```python
from build123d import *

# Parameters (mm, degrees)
EXTRUDE_3_DEPTH     = 5
SKETCH_1_R          = 9.79888
CUT_EXTRUDE_1_DEPTH = 1.65
SKETCH_1_9_R        = 3.15
SKETCH_3_8_R        = 1.65
SKETCH_3_9_R        = 1.648905
SKETCH_3_9_R_2      = 1.65
CUT_EXTRUDE_2_DEPTH = 5
SKETCH_10_R         = 11.19888
CUT_EXTRUDE_3_DEPTH = 3.35
EXTRUDE_4_DEPTH     = 28
EXTRUDE_5_DEPTH     = 2
EXTRUDE_6_DEPTH     = 28


with BuildPart() as part:
    # Sketch 7 → Extrude 3 (new body)
    with BuildSketch(Plane.XY):
        with BuildLine():
            Line((14, 14), (-14, 14))
            Line((-14, 14), (-14, 0))
            ThreePointArc((-14, 0), (-12.934313455, -5.357568053), (-9.899494937, -9.899494937))
            Line((-9.899494937, -9.899494937), (-2.121320344, -17.67766953))
            ThreePointArc((-2.121320344, -17.67766953), (0.000404905, -18.556181469), (2.121892965, -17.677096908))
            Line((2.121892965, -17.677096908), (9.899494937, -9.899494937))
            ThreePointArc((9.899494937, -9.899494937), (12.934313455, -5.357568053), (14, 0))
            Line((14, 0), (14, 14))
        make_face()
    extrude(amount=-EXTRUDE_3_DEPTH)

    # Sketch 1 → Cut-Extrude 1 (cut)
    with BuildSketch(Plane.XY):
        Circle(SKETCH_1_R)
    extrude(amount=-CUT_EXTRUDE_1_DEPTH, mode=Mode.SUBTRACT)

    # Loft 1: read off the stored shape, not the designer's step
    # Loft 1 outline → Loft 1 (revolve, cut)
    with BuildSketch(Plane(origin=(10.6066, 10.606603436, 0), x_dir=(1, 0, 0), z_dir=(0, -1, 0))):
        Polygon((0, 0), (0, -1.5), (1.648905, -1.5), (3.15, 0), align=None)
    revolve(axis=Axis((10.6066, 10.606603436, 0), (0, 0, 1)), mode=Mode.SUBTRACT)

    # Loft 2: read off the stored shape, not the designer's step
    # Loft 2: loft between two sections, ruled curve by curve
    loft_2_from = [
        Edge.make_bspline([(-8.058196468, 12.45812698, 0), (-4.355149378, 7.361319916, 0), (-9.451956443, 3.658272826, 0), (-13.155003532, 8.755079891, 0), (-16.858050622, 13.851886955, 0), (-11.761243557, 17.554934045, 0), (-8.058196468, 12.45812698, 0)], [0, 0, 0, 0, 0.5, 0.5, 0.5, 1, 1, 1, 1], 3, [1, 0.333333333, 0.333333333, 1, 0.333333333, 0.333333333, 1]),
    ]
    loft_2_to = [
        Edge.make_bspline([(-9.518492924, 11.845518562, -1.5), (-7.040662671, 9.669304411, -1.5), (-9.216876823, 7.191474158, -1.5), (-11.694707076, 9.367688309, -1.5), (-14.172537329, 11.543902461, -1.5), (-11.996323177, 14.021732714, -1.5), (-9.518492924, 11.845518562, -1.5)], [0, 0, 0, 0, 0.5, 0.5, 0.5, 1, 1, 1, 1], 3, [1, 0.333333333, 0.333333333, 1, 0.333333333, 0.333333333, 1]),
    ]
    loft_2 = Solid(Shell([*[Face.make_surface_from_curves(loft_2_from[k], loft_2_to[k]) for k in range(1)], Face(Wire(loft_2_from)), Face(Wire(loft_2_to))]))
    add(loft_2, mode=Mode.SUBTRACT)

    # Sketch 1_9 → Loft 3 section 0
    with BuildSketch(Plane.XY):
        with Locations((0, -14.999996564)):
            Circle(SKETCH_1_9_R)
    # Sketch 3_8 → Loft 3 section 1
    with BuildSketch(Plane.XY.offset(-1.5)):
        with Locations((0, -14.999996564)):
            Circle(SKETCH_3_8_R)
    loft(mode=Mode.SUBTRACT)

    # Sketch 3_9 → Cut-Extrude 2 (cut)
    with BuildSketch(Plane.XY.offset(-1.5)):
        with Locations(Location((-10.6066, 10.606603436, 0), (0, 0, 48.708))):
            Circle(SKETCH_3_9_R)
        with Locations((10.6066, 10.606603436)):
            Circle(SKETCH_3_9_R)
        with Locations((0, -14.999996564)):
            Circle(SKETCH_3_9_R_2)
    extrude(amount=-CUT_EXTRUDE_2_DEPTH, mode=Mode.SUBTRACT)

    # Sketch 10 → Cut-Extrude 3 (cut)
    with BuildSketch(Plane(origin=(0, 0, -5), x_dir=(-1, 0, 0), z_dir=(0, 0, -1))):
        Circle(SKETCH_10_R)
    extrude(amount=-CUT_EXTRUDE_3_DEPTH, mode=Mode.SUBTRACT)



with BuildPart() as body_2:
    # Sketch 11 → Extrude 4 (new body)
    with BuildSketch(Plane(origin=(14, 0, 0), x_dir=(0, 0, -1), z_dir=(1, 0, 0))):
        with BuildLine():
            Line((5, 15), (5, 17.5))
            ThreePointArc((5, 17.5), (-2.424621202, 20.575378798), (-5.5, 28))
            Line((-5.5, 28), (-8, 28))
            ThreePointArc((-8, 28), (-4.192388155, 18.807611845), (5, 15))
        make_face()
    extrude(amount=-EXTRUDE_4_DEPTH)

    # Sketch 13 → Extrude 5 (add)
    with BuildSketch(Plane.ZY.offset(-14)):
        with BuildLine():
            Line((-5, 28), (-5, 15))
            ThreePointArc((-5, 15), (4.192388155, 18.807611845), (8, 28))
            Line((8, 28), (-5, 28))
        make_face()
    extrude(amount=EXTRUDE_5_DEPTH)


with BuildPart() as part_1:
    add(part.part)

    add(body_2.part)  # Extrude 6 merges body 2
    # Sketch 14 → Extrude 6 (add)
    with BuildSketch(Plane(origin=(-14, 0, 0), x_dir=(0, 0, -1), z_dir=(1, 0, 0))):
        Polygon((0, 14), (-1.780422928, 16.908297474), (5, 16.908297474), (5, 14), align=None)
    extrude(amount=EXTRUDE_6_DEPTH)


solid = part_1.part
```
For this review, take the finished solid that the model builds, in its own axes (mm). A direction names the side the tool comes from. Round coordinates to 2 decimals unless told otherwise and drop trailing zeros. Write each loop counter-clockwise with the first axis right and the second up, starting at its lowest first coordinate (ties: lowest second). Pieces come first, ordered by that corner, then holes. Notation, with made-up numbers: M 41.25,62 L 83.25,62 A15 ccw 83.25,80 Z; hole C 75,10.5 d3. An arc over 180 degrees is marked long. One line per item, written item: value. Start each with the question number.
(1) We need section C-C (x = -5.75). Give the boundary of the cut face in (y, z).
(2) We need section B-B (x = 0). Give the boundary of the cut face in (y, z), and give its area (3 significant figures).
(3) Insertion check: pin 1 (4 mm diameter, centred on x = 3, y = 9, fed in from -Z); pin 2 (2 mm diameter, centred on x = 3.5, y = 21, fed in from -Z); pin 3 (4.5 mm diameter, centred on x = -10.61, y = 10.61, fed in from +Z); pin 4 (6.5 mm diameter, centred on x = 2.5, y = 4.5, fed in from -Z). Each pin has a flat end and moves straight along its axis. Give the tip position at first contact, or say it passes through.
(4) We need section A-A (y = 2). Give the boundary of the cut face in (x, z), and give its area (3 significant figures).
(5) We need section D-D (z = 4). Give the boundary of the cut face in (x, y).
(6) Machinability: for faces 1 (the flat face through (-6.1, -13.7, -2.5)), 2 (the cylindrical face through (-0.82, 20.49, 2.34)), 3 (the flat face through (10, 0, 0)), which of the approach directions +Z, -Z, +X, -X, +Y, -Y give a long, thin tool a straight path to every point of the face, cutting with its end or side? Answer none if there is none.
(7) The part is to be moulded in two halves that separate along Y. For faces 4 (the flat face through (6, -13.8, -2.5)), 5 (the flat face through (-14, 11, -1)), 6 (the cylindrical face through (1.458, 11.104, -3.348)), say which applies: released by +Y, released by -Y, zero draft, split by the parting line, or undercut.
(8) Wall thickness on line 1 (Y direction, x = 1.5, z = -4); line 2 (Y direction, x = 0, z = -2.4); line 3 (X direction, y = 11.5, z = -2): over which ranges is each line inside the solid? List them lowest first.
Result:
1. outline: M -14.05,-5 L -9.61,-5 L -9.61,-1.65 L -7.93,-1.65 L -7.93,0 L -14.05,0 Z; M 7.93,-1.65 L 9.61,-1.65 L 9.61,-5 L 17.5,-5 A10.5 cw 28,5.5 L 28,8 A13 ccw 16.91,1.78 L 14,0 L 7.93,0 Z
2. outline: M -18.56,-5 L -16.65,-5 L -16.65,-1.5 L -18.15,0 L -18.56,0 Z; M -13.35,-5 L -11.2,-5 L -11.2,-1.65 L -9.8,-1.65 L -9.8,0 L -11.85,0 L -13.35,-1.5 Z; M 9.8,-1.65 L 11.2,-1.65 L 11.2,-5 L 17.5,-5 A10.5 cw 28,5.5 L 28,8 A13 ccw 16.91,1.78 L 14,0 L 9.8,0 Z
2. area: 91.2 mm²
3. pin 1: z = -5
3. pin 2: z = 1.8
3. pin 3: z = -0.88
3. pin 4: through
4. outline: M -14,-5 L -11.02,-5 L -11.02,-1.65 L -9.59,-1.65 L -9.59,0 L -14,0 Z; M 9.59,-1.65 L 11.02,-1.65 L 11.02,-5 L 14,-5 L 14,0 L 9.59,0 Z
4. area: 34.5 mm²
5. outline: M -14,18.62 L 14,18.62 L 14,28 L 12,28 L 12,22.59 L -14,22.59 Z
6. face 1: +Z, -Z, -X, -Y
6. face 2: -Z, -X, +Y
6. face 3: +Z, +X, -X, -Y
7. face 4: released by -Y
7. face 5: zero draft
7. face 6: undercut
8. line 1: -18.15 to -15.69, -14.31 to -11.1, 11.1 to 17.55
8. line 2: -18.56 to -16.65, -13.35 to -11.2, 11.2 to 17.83
8. line 3: -14 to -11.99, -9.22 to 9.22, 11.99 to 14
